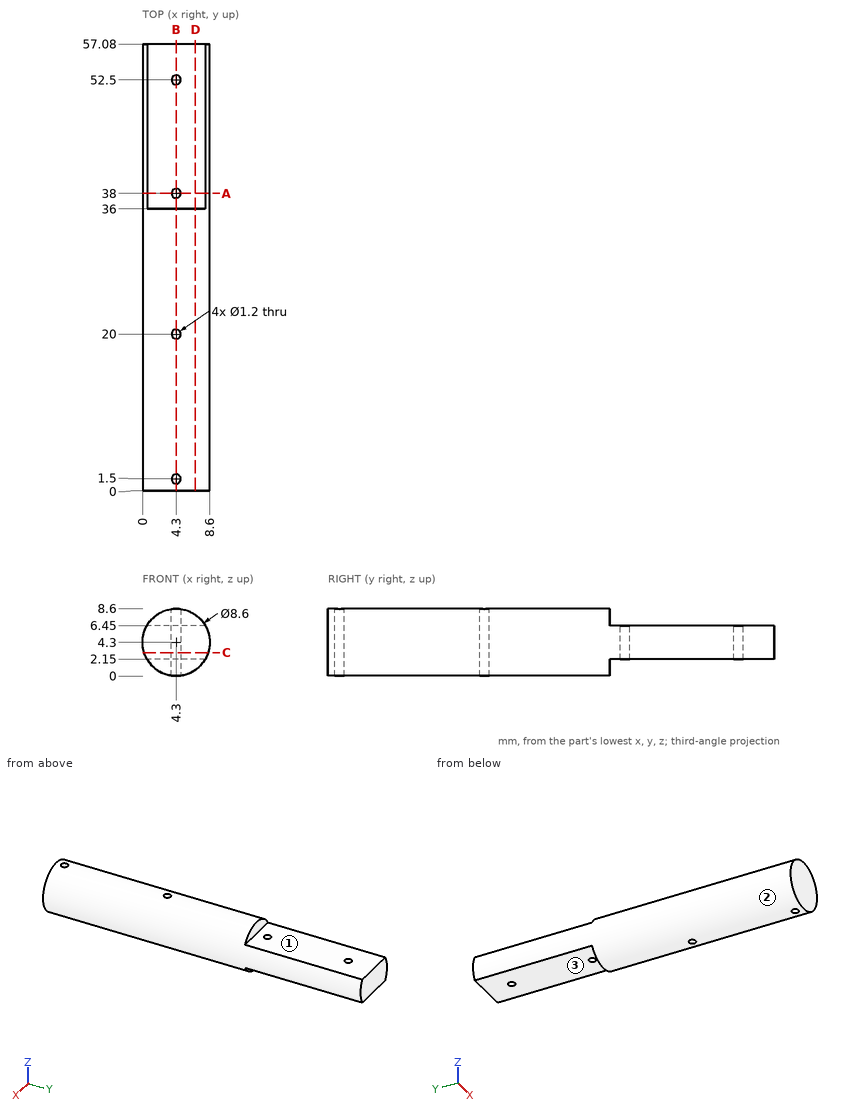
The drawing under review shows one solid part. Ordinate dimensions are in mm from its lowest x, y, z. A direction names the side the tool comes from. Coordinates: 2 decimals unless noted, no trailing zeros. Write each loop counter-clockwise with the first axis right and the second up, starting at its lowest first coordinate (ties: lowest second). Pieces come first, ordered by that corner, then holes. Notation, with made-up numbers: (44.5, -11.5) - (90.5, -11.5) arc R22 cw to (90.5, 16.5) - close; hole circle Ø10 at (39.25, 81.5). An arc over 180 degrees is marked (long way). Answer in a Markdown table with one row per item. Add a question column.
Q1. Tool access review of the marked faces 1, 2 and 3: name each direction out of +Z, -Z, +X, -X, +Y, -Y from which nothing blocks a thin tool from reaching the whole face with its end or side.
Q2. For P1, Ø1.1, axis at x = 4.3, y = 38, coming from the -Z side; P2, Ø3.5, axis at x = 4.5, y = 44.5, coming from the +Z side, all flat-tipped, find the tip position at first contact; note any pin that passes through.
Q3. We need section B-B, the plane x = 4.3. State the section outline as (y, z) points.
Q4. For probe 1 along Y at (x, z) = (4.3, 6.75); probe 2 along Y at (x, z) = (4.3, 6); probe 3 along Z at (x, y) = (6, 52), list the stretches that pass through material, from the lowest coordinate up.
Q5. We need section A-A, the plane y = 38. State the section outline as (x, z) points, and give its area (3 significant figures).
Q6. We need section C-C, the plane z = 3. State the section outline as (x, y) points.
Q7. We need section D-D, the plane x = 6.75. State the section outline as (y, z) points, and give its area (3 significant figures).
Answer list:
| question | item | result |
|---|---|---|
| 1 | face 1 | +Z, +X, -X, +Y |
| 1 | face 2 | +Y, -Y |
| 1 | face 3 | -Z, +X, -X, +Y |
| 2 | P1 | passes through |
| 2 | P2 | stops at z = 6.45 |
| 3 | outline | (0, 0) - (0.9, 0) - (0.9, 8.6) - (0, 8.6) - close; (2.1, 0) - (19.4, 0) - (19.4, 8.6) - (2.1, 8.6) - close; (20.6, 0) - (36, 0) - (36, 2.15) - (37.4, 2.15) - (37.4, 6.45) - (36, 6.45) - (36, 8.6) - (20.6, 8.6) - close; (38.6, 2.15) - (51.9, 2.15) - (51.9, 6.45) - (38.6, 6.45) - close; (53.1, 2.15) - (57.08, 2.15) - (57.08, 6.45) - (53.1, 6.45) - close |
| 4 | probe 1 | y = 0 to 0.9, 2.1 to 19.4, 20.6 to 36 |
| 4 | probe 2 | y = 0 to 0.9, 2.1 to 19.4, 20.6 to 37.4, 38.6 to 51.9, 53.1 to 57.08 |
| 4 | probe 3 | z = 2.15 to 6.45 |
| 5 | outline | (0.58, 2.15) - (3.7, 2.15) - (3.7, 6.45) - (0.58, 6.45) arc R4.3 ccw to start; (4.9, 2.15) - (8.02, 2.15) arc R4.3 ccw to (8.02, 6.45) - (4.9, 6.45) - close |
| 5 | area | 30.2 mm2 |
| 6 | outline | (0.2, 0) - (8.4, 0) - (8.4, 57.08) - (0.2, 57.08) - close; hole circle Ø1.2 at (4.3, 1.5); hole circle Ø1.2 at (4.3, 20); hole circle Ø1.2 at (4.3, 38); hole circle Ø1.2 at (4.3, 52.5) |
| 7 | outline | (0, 0.77) - (36, 0.77) - (36, 2.15) - (57.08, 2.15) - (57.08, 6.45) - (36, 6.45) - (36, 7.83) - (0, 7.83) - close |
| 7 | area | 345 mm2 |
